Study the drawing (mm; zero at the part's minimum x, y, z) and answer. A direction names the side the tool comes from. Round coordinates to 2 decimals unless told otherwise and drop trailing zeros. Write each loop counter-clockwise with the first axis right and the second up, starting at its lowest first coordinate (ties: lowest second). Pieces come first, ordered by that corner, then holes. Notation, with made-up numbers: (7.25, 61) - (47.25, 61) arc R21 cw to (47.25, 90) - close; hole circle Ø3 at (31.25, 35). An arc over 180 degrees is marked (long way). Use one line per item in the form item = value. Start each with the question number.
1) Consider line 1 along Y through (x, z) = (3, 8); line 2 along Y through (x, z) = (7.5, 3.5). Determine where each line is inside the solid, lowest interval first. Write a range as from..to.
2) The part is cut by section A-A, the plane z = 6. Give the vertices of the cut face in (x, y).
3) For a pull along X with two mould halves and no side action, classify the marked faces 1, 2, 3 and 4 as released by +X, released by -X, zero draft, split by the parting line, or undercut.
4) Each of these flat-tipped pins is pushed along its axis until it touches: pin 1 (3 mm diameter, centred on x = 7.5, z = 7.5, fed in from +Y); pin 2 (4.5 mm diameter, centred on x = 17.5, z = 6.5, fed in from -Y); pin 3 (4.5 mm diameter, centred on y = 17.5, z = 6, fed in from -X). Where does it stop, or does it pass through?
5) For the marked faces 5, 6, 7, 8 and 9, determine the directions among +Z, -Z, +X, -X, +Y, -Y from which every point of the face is accessible in a straight line to the end or side of a thin tool.
6) The part is cut by section B-B, the plane x = 18. Give the vertices of the cut face in (y, z), plus the area to 3 significant figures.
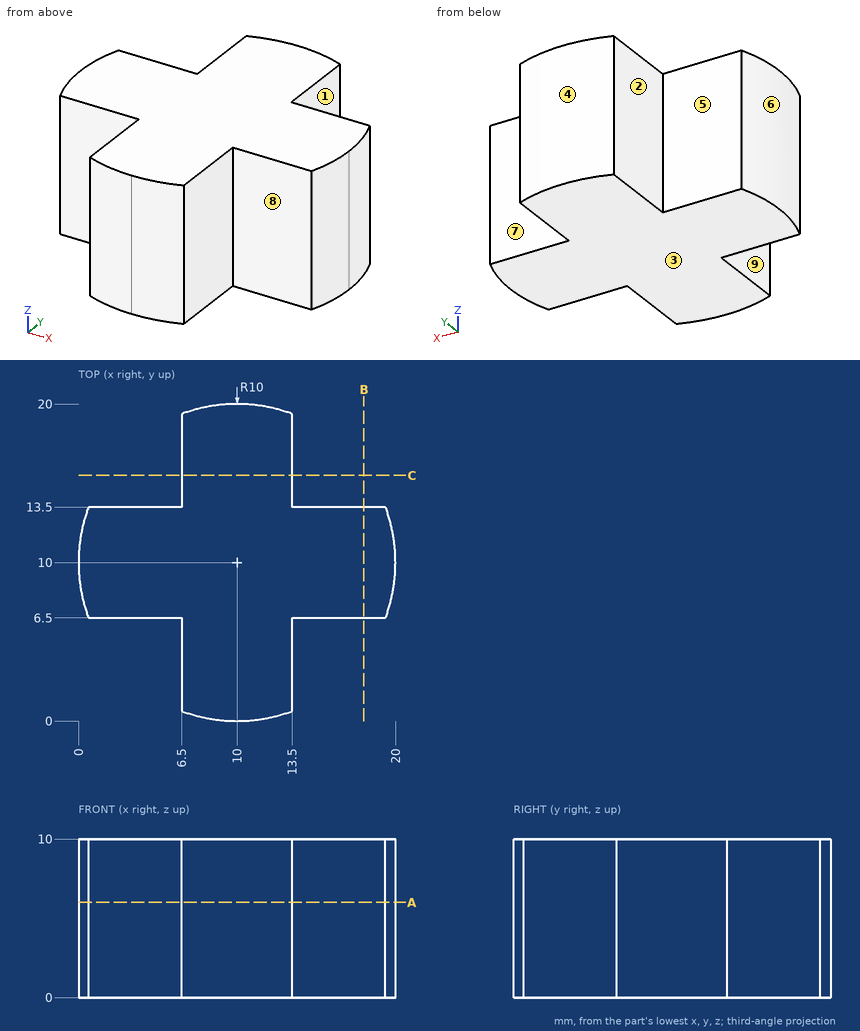
Geometry results:
q1.line_1 = 6.5..13.5
q1.line_2 = 0.32..19.68
q2.outline = (0.63, 6.5) - (6.5, 6.5) - (6.5, 0.63) arc R10 ccw to (13.5, 0.63) - (13.5, 6.5) - (19.37, 6.5) arc R10 ccw to (19.37, 13.5) - (13.5, 13.5) - (13.5, 19.37) arc R10 ccw to (6.5, 19.37) - (6.5, 13.5) - (0.63, 13.5) arc R10 ccw to start
q3.face_1 = released by +X
q3.face_2 = released by -X
q3.face_3 = zero draft
q3.face_4 = split by the parting line
q4.pin_1 = 19.95
q4.pin_2 = 6.5
q4.pin_3 = 6.5
q5.face_5 = +Z, -Z, -X, +Y
q5.face_6 = +Z, -Z, -X
q5.face_7 = +Z, -Z, +X, +Y
q5.face_8 = +Z, -Z, +X, -Y
q5.face_9 = +Z, -Z, -X, -Y
q6.outline = (6.5, 0) - (13.5, 0) - (13.5, 10) - (6.5, 10) - close
q6.area = 70.0 mm2
